Input: dimensioned drawing with shaded views. Units: mm. Origin: part minimum x, y, z. Give positions to 0.01 mm unless a question says otherwise; leave off trailing zeros. Write each loop counter-clockwise with the first axis right and the second up, starting at its lowest first coordinate (ties: lowest second). Pieces come first, ordered by that corner, then holes. Notation, with made-up numbers: (39, -14) -> (62, -14) arc R11 ccw to (62, 0) -> close; hole circle Ø3 at (-23.75, 35.5). An arc over 180 degrees is marked (long way). Return JSON: item names as keys, results as strings. Group by question number.
Item 1: Mould query, pull axis X, two halves, no side actions, for the marked faces 1, 2 and 3. Classes: released by +X, released by -X, zero draft, split by the parting line, or undercut.
Item 2: Section C-C, the plane x = 6.5. Return loops of the section in (y, z).
Item 3: Line query: line 1 (Z direction, x = 8.75, y = 0.25); line 2 (X direction, y = 1.7, z = 0.8); line 3 (Y direction, x = 1.25, z = 0.85). Output: solid intervals per line, ascending. Write a range as [from, to].
Item 4: Section A-A, the plane z = 1.75. Return loops of the section in (x, y) (1 decimal).
Item 5: Section D-D, the plane z = 0.7. Return loops of the section in (x, y).
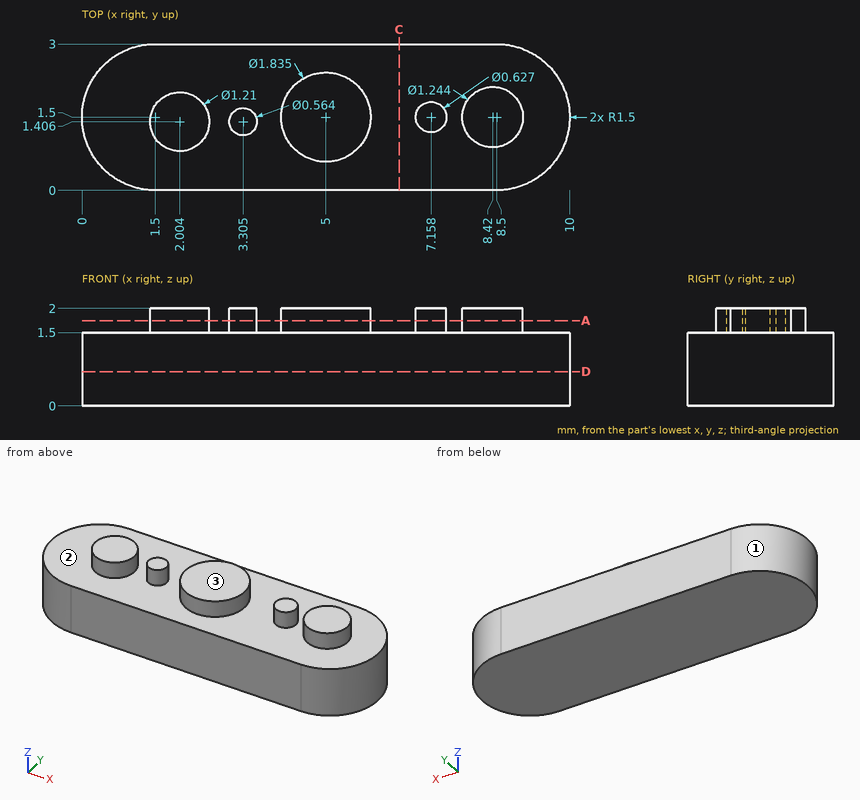
Answer below:
{
 "1": {"face 1": "released by -X", "face 2": "undercut", "face 3": "zero draft"},
 "2": {"outline": "(0, 0) -> (3, 0) -> (3, 1.5) -> (0, 1.5) -> close"},
 "3": {"line 1": "z = [0, 1.5]", "line 2": "x = [0.01, 9.99]", "line 3": "y = [0.02, 2.98]"},
 "4": {"outline": "circle Ø1.2 at (2, 1.4); circle Ø0.6 at (3.3, 1.4); circle Ø1.8 at (5, 1.5); circle Ø0.6 at (7.2, 1.5); circle Ø1.2 at (8.4, 1.5)"},
 "5": {"outline": "(1.5, 0) -> (8.5, 0) arc R1.5 ccw to (8.5, 3) -> (1.5, 3) arc R1.5 ccw to start"}
}
